```python
from build123d import *

# Parameters (mm, degrees)
SKETCH1_R               = 2.65
BOSS_EXTRUDE1_DEPTH     = 69.85
BOSS_EXTRUDE2_REACH     = 119.557
BOSS_EXTRUDE3_REACH     = 116.246
CUT_EXTRUDE3_START      = -35.94
SKETCH7_R               = 2.65
CUT_EXTRUDE3_DEPTH      = 23.24
CUT_EXTRUDE2_START      = -12.7
SKETCH6_R               = 2.65
CUT_EXTRUDE2_DEPTH      = 44.45
FILLET1_R               = 0.508
SKETCH8_W               = 20
SKETCH8_H               = 20
CUT_EXTRUDE4_DEPTH      = 3.5
CUT_EXTRUDE6_DEPTH      = 117.039655722
CUT_EXTRUDE6_DEPTH_BACK = 117.039655722
SKETCH10_R              = 1.5
SKETCH10_W              = 4.926728391
SKETCH10_H              = 20


with BuildPart() as part:
    # Sketch1 → Boss-Extrude1 (new body)
    with BuildSketch(Plane(origin=(0, 0, 0), x_dir=(1, 0, 0), z_dir=(0, 1, 0))):
        with BuildLine():
            ThreePointArc((55.958719807, -7.48245925), (69.572262573, -2.613222795), (60.96, 9))
            Line((60.96, 9), (54.61, 9))
            Line((54.61, 9), (54.61, 45.61))
            Line((54.61, 45.61), (60.96, 45.61))
            ThreePointArc((60.96, 45.61), (69.27112045, 58.063299416), (54.582047244, 60.959938476))
            Line((54.582047244, 60.959938476), (48.26, 54.61))
            Line((48.26, 54.61), (48.26, 6.35))
            Line((48.26, 6.35), (0, 6.35))
            Line((0, 6.35), (0, 0))
            Line((0, 0), (48.26, 0))
            Line((48.26, 0), (55.958719807, -7.48245925))
        make_face()
        with Locations(Location((60.96, 0, 0), (0, 0, 270))):
            Circle(SKETCH1_R, mode=Mode.SUBTRACT)
        with Locations(Location((60.96, 54.61, 0), (0, 0, 270))):
            Circle(SKETCH1_R, mode=Mode.SUBTRACT)
    extrude(amount=BOSS_EXTRUDE1_DEPTH)

    # Sketch3 → Boss-Extrude2 (add, up to next)
    with BuildSketch(Plane.ZY, mode=Mode.PRIVATE) as boss_extrude2_sk1:
        Polygon((-6.35, 69.85), (-6.35, 63.5), (-12.7, 69.85), align=None)
    boss_extrude2_tool1 = extrude(boss_extrude2_sk1.sketch, amount=-BOSS_EXTRUDE2_REACH, mode=Mode.PRIVATE) - part.part
    # Sketch3 → Boss-Extrude2 (add, up to next)
    with BuildSketch(Plane.ZY, mode=Mode.PRIVATE) as boss_extrude2_sk2:
        Polygon((-6.35, 0), (-6.35, 6.35), (-12.7, 0), align=None)
    boss_extrude2_tool2 = extrude(boss_extrude2_sk2.sketch, amount=-BOSS_EXTRUDE2_REACH, mode=Mode.PRIVATE) - part.part
    add(boss_extrude2_tool1.solids().sort_by_distance((0, 67.733333, -8.466667))[0])
    add(boss_extrude2_tool2.solids().sort_by_distance((0, 2.116667, -8.466667))[0])

    # Boss-Extrude3: up to this plane
    boss_extrude3_end = Plane(origin=(-3.068514972, 69.85, -3.055036942), z_dir=(-0.7086614173228347, 0, -0.7055487195070168))
    # Sketch4 → Boss-Extrude3 (add, up to the surface)
    with BuildSketch(Plane(origin=(0, 0, -6.35), x_dir=(-1, 0, 0), z_dir=(0, 0, -1)), mode=Mode.PRIVATE) as boss_extrude3_sk1:
        Polygon((-48.26, 69.85), (-48.26, 63.5), (-41.91, 69.85), align=None)
    boss_extrude3_tool1 = split(extrude(boss_extrude3_sk1.sketch, amount=BOSS_EXTRUDE3_REACH, mode=Mode.PRIVATE), bisect_by=boss_extrude3_end, keep=Keep.BOTH, mode=Mode.PRIVATE)
    add(boss_extrude3_tool1.solids().sort_by_distance((46.143333, 67.733333, -6.35))[0])
    # Sketch4 → Boss-Extrude3 (add, up to the surface)
    with BuildSketch(Plane(origin=(0, 0, -6.35), x_dir=(-1, 0, 0), z_dir=(0, 0, -1)), mode=Mode.PRIVATE) as boss_extrude3_sk2:
        Polygon((-48.26, 6.35), (-48.26, 0), (-41.91, 0), align=None)
    boss_extrude3_tool2 = split(extrude(boss_extrude3_sk2.sketch, amount=BOSS_EXTRUDE3_REACH, mode=Mode.PRIVATE), bisect_by=boss_extrude3_end, keep=Keep.BOTH, mode=Mode.PRIVATE)
    add(boss_extrude3_tool2.solids().sort_by_distance((46.143333, 2.116667, -6.35))[0])

    # Sketch7 → Cut-Extrude3 (cut)
    # profile 1 of 4: a face of its own
    with BuildSketch(Plane(origin=(0, 69.85, 0), x_dir=(1, 0, 0), z_dir=(0, 1, 0)).offset(CUT_EXTRUDE3_START)):
        with BuildLine():
            ThreePointArc((52.001434215, 53.747388227), (52.824115031, 50.761964686), (54.61, 48.232108499))
            ThreePointArc((54.61, 48.232108499), (57.524961682, 46.291315503), (60.96, 45.61))
            ThreePointArc((60.96, 45.61), (67.323961031, 48.246038969), (69.96, 54.61))
            ThreePointArc((69.96, 54.61), (64.394998195, 62.928701065), (54.582047244, 60.959938476))
            ThreePointArc((54.582047244, 60.959938476), (52.641298935, 58.044998195), (51.96, 54.61))
            ThreePointArc((51.96, 54.61), (51.970364522, 54.178196843), (52.001434215, 53.747388227))
        make_face()
        with Locations(Location((60.96, 54.61, 0), (0, 0, 270))):
            Circle(SKETCH7_R, mode=Mode.SUBTRACT)
    # profile 2 of 4: a face of its own
    with BuildSketch(Plane(origin=(0, 69.85, 0), x_dir=(1, 0, 0), z_dir=(0, 1, 0)).offset(CUT_EXTRUDE3_START)):
        with BuildLine():
            Line((54.61, 48.232108499), (54.61, 45.61))
            Line((54.61, 45.61), (60.96, 45.61))
            ThreePointArc((60.96, 45.61), (57.524961682, 46.291315503), (54.61, 48.232108499))
        make_face()
    # profile 3 of 4: a face of its own
    with BuildSketch(Plane(origin=(0, 69.85, 0), x_dir=(1, 0, 0), z_dir=(0, 1, 0)).offset(CUT_EXTRUDE3_START)):
        with BuildLine():
            Line((51.96, 58.32632344), (51.96, 54.61))
            ThreePointArc((51.96, 54.61), (52.641298935, 58.044998195), (54.582047244, 60.959938476))
            Line((54.582047244, 60.959938476), (51.96, 58.32632344))
        make_face()
    # profile 4 of 4: a face of its own
    with BuildSketch(Plane(origin=(0, 69.85, 0), x_dir=(1, 0, 0), z_dir=(0, 1, 0)).offset(CUT_EXTRUDE3_START)):
        with BuildLine():
            Line((54.61, 26.656396737), (54.61, 45.61))
            Line((54.61, 45.61), (54.61, 48.232108499))
            ThreePointArc((54.61, 48.232108499), (52.824115031, 50.761964686), (52.001434215, 53.747388227))
            Line((52.001434215, 53.747388227), (54.61, 26.656396737))
        make_face()
    extrude(amount=CUT_EXTRUDE3_DEPTH, mode=Mode.SUBTRACT)

    # Sketch6 → Cut-Extrude2 (cut)
    # profile 1 of 7: a face of its own
    with BuildSketch(Plane(origin=(0, 0, 0), x_dir=(-1, 0, 0), z_dir=(0, -1, 0)).offset(CUT_EXTRUDE2_START)):
        with BuildLine():
            Line((-60.96, 9), (-57.841406567, 9))
            ThreePointArc((-57.841406567, 9), (-69.785888373, -3.581803934), (-52.451441296, -4.281361207))
            ThreePointArc((-52.451441296, -4.281361207), (-52.357529126, -4.089391135), (-52.267947508, -3.895362431))
            Line((-52.267947508, -3.895362431), (-55.958719807, -7.48245925))
            ThreePointArc((-55.958719807, -7.48245925), (-69.572262573, -2.613222795), (-60.96, 9))
        make_face()
    # profile 2 of 7: a face of its own
    with BuildSketch(Plane(origin=(0, 0, 0), x_dir=(-1, 0, 0), z_dir=(0, -1, 0)).offset(CUT_EXTRUDE2_START)):
        with BuildLine():
            ThreePointArc((-53.816250004, 6.300195314), (-54.20129816, 6.711599991), (-54.61, 7.099515829))
            ThreePointArc((-54.61, 7.099515829), (-56.131281182, 8.210304475), (-57.841406567, 9))
            Line((-57.841406567, 9), (-60.96, 9))
            ThreePointArc((-60.96, 9), (-69.572262573, -2.613222795), (-55.958719807, -7.48245925))
            Line((-55.958719807, -7.48245925), (-52.267947508, -3.895362431))
            ThreePointArc((-52.267947508, -3.895362431), (-51.645564295, -1.991710949), (-51.435, 0))
            ThreePointArc((-51.435, 0), (-52.050178349, 3.367596048), (-53.816250004, 6.300195314))
        make_face()
        with Locations(Location((-60.96, 0, 0), (0, 0, 270))):
            Circle(SKETCH6_R, mode=Mode.SUBTRACT)
    # profile 3 of 7: a face of its own
    with BuildSketch(Plane(origin=(0, 0, 0), x_dir=(-1, 0, 0), z_dir=(0, -1, 0)).offset(CUT_EXTRUDE2_START)):
        with Locations(Location((-60.96, 0, 0), (0, 0, 270))):
            Circle(SKETCH6_R)
    # profile 4 of 7: a face of its own
    with BuildSketch(Plane(origin=(0, 0, 0), x_dir=(-1, 0, 0), z_dir=(0, -1, 0)).offset(CUT_EXTRUDE2_START)):
        with BuildLine():
            Line((-52.267947508, -3.895362431), (-48.26, 0))
            Line((-48.26, 0), (-51.435, 0))
            ThreePointArc((-51.435, 0), (-51.645564295, -1.991710949), (-52.267947508, -3.895362431))
        make_face()
    # profile 5 of 7: a face of its own
    with BuildSketch(Plane(origin=(0, 0, 0), x_dir=(-1, 0, 0), z_dir=(0, -1, 0)).offset(CUT_EXTRUDE2_START)):
        with BuildLine():
            ThreePointArc((-52.267947508, -3.895362431), (-52.357529126, -4.089391135), (-52.451441296, -4.281361207))
            Line((-52.451441296, -4.281361207), (-48.26, 0))
            Line((-48.26, 0), (-52.267947508, -3.895362431))
        make_face()
    # profile 6 of 7: a face of its own
    with BuildSketch(Plane(origin=(0, 0, 0), x_dir=(-1, 0, 0), z_dir=(0, -1, 0)).offset(CUT_EXTRUDE2_START)):
        with BuildLine():
            Line((-54.61, 7.099515829), (-54.61, 9))
            Line((-54.61, 9), (-57.841406567, 9))
            ThreePointArc((-57.841406567, 9), (-56.131281182, 8.210304475), (-54.61, 7.099515829))
        make_face()
    # profile 7 of 7: a face of its own
    with BuildSketch(Plane(origin=(0, 0, 0), x_dir=(-1, 0, 0), z_dir=(0, -1, 0)).offset(CUT_EXTRUDE2_START)):
        with BuildLine():
            Line((-48.26, 0), (-53.816250004, 6.300195314))
            ThreePointArc((-53.816250004, 6.300195314), (-52.050178349, 3.367596048), (-51.435, 0))
            Line((-51.435, 0), (-48.26, 0))
        make_face()
    extrude(amount=-CUT_EXTRUDE2_DEPTH, mode=Mode.SUBTRACT)

    # Fillet1
    fillet1_edges = [part.edges().sort_by_distance(p)[0] for p in [
        (20.955, 69.85, -12.7),
        (41.91, 69.85, -30.465992724),
        (20.955, 0, -12.7),
        (41.91, 0, -30.465992724),
    ]]
    fillet(fillet1_edges, radius=FILLET1_R)

    # Sketch8 → Cut-Extrude4 (cut)
    with BuildSketch(Plane(origin=(0, 0, -6.35), x_dir=(-1, 0, 0), z_dir=(0, 0, -1))):
        with Locations((-22.385, 38.1)):
            Rectangle(SKETCH8_W, SKETCH8_H)
    extrude(amount=-CUT_EXTRUDE4_DEPTH, mode=Mode.SUBTRACT)

    # Sketch10 → Cut-Extrude6 (cut, two sides: drawn at the far end of the back side and taken through both)
    with BuildSketch(Plane(origin=(0, 0, -2.85), x_dir=(-1, 0, 0), z_dir=(0, 0, -1)).offset(-CUT_EXTRUDE6_DEPTH_BACK)):
        with Locations((-14.885, 30.6)):
            Circle(SKETCH10_R)
        with Locations((-14.885, 45.6)):
            Circle(SKETCH10_R)
        with Locations((-29.921635805, 38.1)):
            Rectangle(SKETCH10_W, SKETCH10_H)
    extrude(amount=CUT_EXTRUDE6_DEPTH + CUT_EXTRUDE6_DEPTH_BACK, mode=Mode.SUBTRACT)


solid = part.part
```
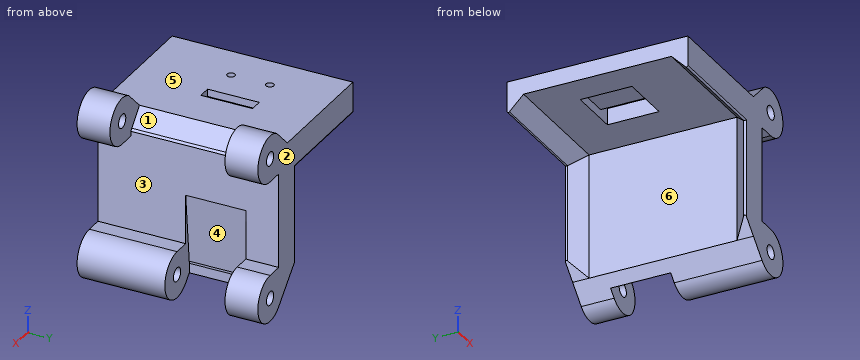
Can you work these out from the model? Positions are in its coordinate system, mm. Face numbers are marked on the shaded views. A direction names the side the tool comes from. Give positions to 0.01 mm unless a question says otherwise; leave off trailing zeros. Write each loop counter-clockwise with the first axis right and the second up, starting at its lowest first coordinate (ties: lowest second). Pieces come first, ordered by that corner, then holes. Notation, with made-up numbers: (66.5, 89.25) -> (85.5, 89.25) arc R32 ccw to (85.5, 126.25) -> close; hole circle Ø10 at (80.25, -2.75). An arc over 180 degrees is marked (long way). Write item = value, one per line.
(1) I need wall thicknesses on probe 1 along Y at (x, z) = (61, -60); probe 2 along Z at (x, y) = (7.5, 22); probe 3 along X at (y, z) = (24, -22). Which ranges of each line are inside material? Lowest first, please. Write a range as from..to.
Worked out:
probe_1 = 0..33.91, 57.15..69.85
probe_2 = -6.35..0
probe_3 = 48.26..54.61
(2) Suppose I cut it at B-B on y = 39.5. Write out the boundary of the cut face in (x, z) (3 decimals), then the cut area to 3 significant figures.
Worked out:
outline = (0, -6.35) -> (12.385, -6.35) -> (12.385, -2.85) -> (27.458, -2.85) -> (27.458, 0) -> (0, 0) -> close; (32.385, -6.35) -> (48.26, -6.35) -> (48.26, -54.61) -> (51.96, -58.326) -> (51.96, -54.61) arc R9 cw to (52.001, -53.747) -> (54.61, -26.656) -> (54.61, -7.1) arc R9.525 cw to (53.816, -6.3) -> (48.26, 0) -> (32.385, 0) -> close
area = 516 mm^2
(3) Thinking about a two-plate mould opening in Z: for the marked faces 1, 2 and 3, which applies, released by +Z, released by -Z, zero draft, split by the parting line, or undercut?
Worked out:
face_1 = released by +Z
face_2 = zero draft
face_3 = undercut
(4) Suppose I cut it at D-D on z = -4.5. Write out the boundary of the cut face in (x, y) (3 decimals).
Worked out:
outline = (0, 0) -> (68.754, 0) -> (68.754, 12.7) -> (52.229, 12.7) -> (52.229, 57.15) -> (68.754, 57.15) -> (68.754, 69.85) -> (0, 69.85) -> close; hole (12.385, 28.1) -> (32.385, 28.1) -> (32.385, 48.1) -> (12.385, 48.1) -> close
(5) Suppose I cut it at C-C on y = 20. Write out the boundary of the cut face in (x, z) (3 decimals), then the cut area to 3 significant figures.
Worked out:
outline = (0, -6.35) -> (48.26, -6.35) -> (48.26, -54.61) -> (54.582, -60.96) arc R9 ccw (long way) to (60.96, -45.61) -> (54.61, -45.61) -> (54.61, -7.1) arc R9.525 cw to (53.816, -6.3) -> (48.26, 0) -> (0, 0) -> close; hole circle Ø5.3 at (60.96, -54.61)
area = 865 mm^2
(6) I'm going to push flat-ended pins straight in: P1, Ø1.9, axis at x = 58.5, y = 64.5, coming from the -Z side; P2, Ø1.9, axis at x = 57, y = 13, coming from the +Z side; P3, Ø7, axis at x = 60.96, z = -54.61, coming from the -Y side; P4, Ø10, axis at y = 39, z = -54, coming from the +X side. Where does each tip first touch, or does it pass through?
Worked out:
P1 = -63.48
P2 = 8.46
P3 = 0
P4 = 52.46
(7) For the marked faces 4, 5 and 6, which set-ups out of +Z, -Z, +X, -X, +Y, -Y let a thin tool reach every point of the face, with its end or its side?
Worked out:
face_4 = -Z, +X
face_5 = +Z, -X, +Y, -Y
face_6 = -Z, -X
(8) Suppose I cut it at A-A on y = 30.6. Write out the boundary of the cut face in (x, z) (3 decimals).
Worked out:
outline = (0, -6.35) -> (12.385, -6.35) -> (12.385, -2.85) -> (13.385, -2.85) -> (13.385, 0) -> (0, 0) -> close; (16.385, -2.85) -> (27.458, -2.85) -> (27.458, 0) -> (16.385, 0) -> close; (32.385, -6.35) -> (48.26, -6.35) -> (48.26, -54.61) -> (54.582, -60.96) arc R9 ccw (long way) to (60.96, -45.61) -> (54.61, -45.61) -> (54.61, -7.1) arc R9.525 cw to (53.816, -6.3) -> (48.26, 0) -> (32.385, 0) -> close; hole circle Ø5.3 at (60.96, -54.61)
